```python
from build123d import *

# Parameters (mm, degrees)
SKETCH1_R           = 68.659375
SKETCH1_R_2         = 55.959375
BOSS_EXTRUDE1_DEPTH = 3.175
BOSS_EXTRUDE2_START = -3.175
BOSS_EXTRUDE2_DEPTH = 3.175
CIRPATTERN1_COUNT   = 9
SKETCH3_R           = 2.2225
CUT_EXTRUDE6_DEPTH  = 124.199501286
CIRPATTERN10_COUNT  = 9
CUT_EXTRUDE7_DEPTH  = 124.199501286
CIRPATTERN12_COUNT  = 9
FILLET1_R           = 5.08


with BuildPart() as part:
    # Sketch1 → Boss-Extrude1 (new body)
    with BuildSketch(Plane(origin=(0, 0, 0), x_dir=(1, 0, 0), z_dir=(0, 1, 0))):
        with Locations(Location((0, 0, 0), (0, 0, 270))):
            Circle(SKETCH1_R)
        with Locations(Location((0, 0, 0), (0, 0, 270))):
            Circle(SKETCH1_R_2, mode=Mode.SUBTRACT)
    extrude(amount=BOSS_EXTRUDE1_DEPTH)

    # Sketch2 → Boss-Extrude2 (add)
    with BuildSketch(Plane(origin=(0, 3.175, 0), x_dir=(1, 0, 0), z_dir=(0, 1, 0)).offset(BOSS_EXTRUDE2_START)):
        with BuildLine():
            Line((-4.653697789, 71.001707707), (-5.372788209, 81.972907412))
            ThreePointArc((-5.372788209, 81.972907412), (0, 87.709375), (5.372788209, 81.972907412))
            ThreePointArc((5.372788209, 81.972907412), (1.580107525, 80.725221164), (0.983574692, 76.777399446))
            Line((0.983574692, 76.777399446), (3.889375, 69.933810414))
            ThreePointArc((3.889375, 69.933810414), (4.734169071, 68.871766239), (6.005193091, 68.39625305))
            ThreePointArc((6.005193091, 68.39625305), (-0.46538454, 68.657797755), (-6.931822104, 68.308561818))
            ThreePointArc((-6.931822104, 68.308561818), (-5.249012804, 69.195180628), (-4.653697789, 71.001707707))
        make_face()
    boss_extrude2 = extrude(amount=BOSS_EXTRUDE2_DEPTH)

    # CirPattern1: Boss-Extrude2 ×9 about axis
    cirpattern1_axis = Axis((0, 0, 0), (0, 1, 0))
    for i in range(1, CIRPATTERN1_COUNT):
        add(boss_extrude2.rotate(cirpattern1_axis, i * 360 / CIRPATTERN1_COUNT))

    # Sketch3 → Cut-Extrude6 (cut, through all)
    with BuildSketch(Plane(origin=(0, 3.175, 0), x_dir=(1, 0, 0), z_dir=(0, 1, 0))):
        with Locations(Location((0, 84.132166, 0), (0, 0, 270))):
            Circle(SKETCH3_R)
    cut_extrude6 = extrude(amount=-CUT_EXTRUDE6_DEPTH, mode=Mode.SUBTRACT)

    # CirPattern10: Cut-Extrude6 ×9 about axis
    cirpattern10_axis = Axis((0, 0, 0), (0, 1, 0))
    for i in range(1, CIRPATTERN10_COUNT):
        add(cut_extrude6.rotate(cirpattern10_axis, i * 360 / CIRPATTERN10_COUNT), mode=Mode.SUBTRACT)

    # Sketch4 → Cut-Extrude7 (cut, through all)
    with BuildSketch(Plane(origin=(0, 3.175, 0), x_dir=(1, 0, 0), z_dir=(0, 1, 0))):
        with BuildLine():
            Line((18.267202623, 60.462203187), (6.005193091, 68.39625305))
            ThreePointArc((6.005193091, 68.39625305), (23.04503141, 64.676396797), (38.597813369, 56.78308356))
            Line((38.597813369, 56.78308356), (24.870866002, 58.05866628))
            ThreePointArc((24.870866002, 58.05866628), (21.122906044, 58.034707389), (18.267202623, 60.462203187))
        make_face()
    cut_extrude7 = extrude(amount=-CUT_EXTRUDE7_DEPTH, mode=Mode.SUBTRACT)

    # CirPattern12: Cut-Extrude7 ×9 about axis
    cirpattern12_axis = Axis((0, 0, 0), (0, 1, 0))
    for i in range(1, CIRPATTERN12_COUNT):
        add(cut_extrude7.rotate(cirpattern12_axis, i * 360 / CIRPATTERN12_COUNT), mode=Mode.SUBTRACT)

    # Fillet1
    fillet1_edges = [part.edges().sort_by_distance(p)[0] for p in [
        (-16.849122023, 1.5875, 66.559874267),
        (-62.235489211, 1.5875, 28.997476754),
        (-55.691038779, 1.5875, 40.157414946),
        (6.005193091, 1.5875, -68.39625305),
        (-66.314369444, 1.5875, -17.790845415),
        (-68.474499552, 1.5875, -5.035145128),
        (-6.931822104, 1.5875, -68.308561818),
        (-39.364019213, 1.5875, -56.254633292),
        (-49.217980976, 1.5875, -47.871704837),
        (24.870866002, 1.5875, -58.05866628),
        (18.267202623, 1.5875, -60.462203187),
        (56.371580016, 1.5875, -28.48883417),
        (52.857844124, 1.5875, -34.574803261),
        (61.49540524, 1.5875, 14.411240066),
        (62.715712909, 1.5875, 7.490531368),
        (37.844846907, 1.5875, 50.568134912),
        (43.228202617, 1.5875, 46.050963121),
        (-3.513735893, 1.5875, 63.063637431),
        (3.513735893, 1.5875, 63.063637431),
        (-43.228202617, 1.5875, 46.050963121),
        (-37.844846907, 1.5875, 50.568134912),
        (-62.715712909, 1.5875, 7.490531368),
        (-61.49540524, 1.5875, 14.411240066),
        (-52.857844124, 1.5875, -34.574803261),
        (-56.371580016, 1.5875, -28.48883417),
        (-18.267202623, 1.5875, -60.462203187),
        (-24.870866002, 1.5875, -58.05866628),
        (48.564508807, 1.5875, -48.534505867),
        (38.597813369, 1.5875, -56.78308356),
        (68.399951118, 1.5875, -5.962923987),
        (66.067103, 1.5875, -18.68816943),
        (56.23029612, 1.5875, 39.398776296),
        (62.622860883, 1.5875, 28.151146872),
        (17.749860638, 1.5875, 66.325351282),
        (29.876686184, 1.5875, 61.818228688),
        (-29.035931905, 1.5875, 62.217557279),
    ]]
    fillet(fillet1_edges, radius=FILLET1_R)


solid = part.part
```
Here's how the part is built. I have some questions about the finished solid (model axes, mm). A direction names the side the tool comes from. Coordinates: 2 decimals unless noted, no trailing zeros. Loops run counter-clockwise (first coordinate to the right, second up) from the corner with the lowest first, then second, coordinate; pieces in that order, holes last. Notation, with made-up numbers: (51.5, 1) - (109.5, 1) arc R27 cw to (109.5, 39) - close; hole circle Ø3 at (29, -32). An arc over 180 degrees is marked (long way). Return JSON: item names as keys, results as strings. Group by question number.
Item 1: On a 3-axis mill with a long thin cutter (end or side, diameter ignored), from which of +Z, -Z, +X, -X, +Y, -Y can I reach the whole of each face in a straight line? I mean faces 1 (the face through (-65.636, 1.61, 1.139)), 2 (the face through (30.84, 1.57, 70.09)), 3 (the face through (22.835, 1.565, 69.803)), 4 (the face through (45.279, 1.565, -61.753)). Say none if no direction works.
Item 2: If we section it at B-B on y = 2.25: State how many separate pieces and enclosed holes the cut face has, and give its area (3 significant figures).
Item 3: Will this pin go through, and if not, where does the flat tip stop? P1, Ø1.5, axis at y = 0.5, z = -42, coming from the -X side.
Item 4: If we section it at A-A on z = 0: Write out the boundary of the cut face in (x, y) (3 decimals).
Item 5: If we section it at C-C on z = -25.5: Write out the boundary of the cut face in (x, y) (3 decimals), and give its area (3 significant figures).
Item 6: I need wall thicknesses on line 1 (Z direction, x = 25.5, y = 2.7); line 2 (X direction, y = 0.6, z = -14); line 3 (X direction, y = 0.9, z = 42.5). Which ranges of each line are inside material? Lowest first, please. Write a range as from..to.
Item 7: We'd pull the mould along X, two halves only. Please class faces 5 (the face through (39.65, 1.61, 47.35)), 6 (the face through (-38, 0, 41.3)), 7 (the face through (50.72, 1.61, -41.53)): +X half, -X half, draft (parallel to the pull), parting line (faces both ways), or undercut.
Calculated:
{
 "1": {"face 1": "-X, +Y, -Y", "face 2": "+X, +Y, -Y", "face 3": "+Y, -Y", "face 4": "-Z, +Y, -Y"},
 "2": {"separate pieces": "1", "enclosed holes": "10", "area": "4,990 mm^2"},
 "3": {"P1": "stops at x = -51.03"},
 "4": {"outline": "(-66.16, 0) - (-55.959, 0) - (-55.959, 3.175) - (-66.16, 3.175) - close; (55.959, 0) - (65.881, 0) - (65.881, 3.175) - (55.959, 3.175) - close"},
 "5": {"outline": "(-59.149, 0) - (-49.812, 0) - (-49.812, 3.175) - (-59.149, 3.175) - close; (49.812, 0) - (59.328, 0) - (59.328, 3.175) - (49.812, 3.175) - close", "area": "59.9 mm^2"},
 "6": {"line 1": "z = -57.99..-49.81, 49.81..72.67, 77.49..82.04", "line 2": "x = -86.45..-84.99, -80.72..-54.18, 54.18..80.72, 84.99..86.45", "line 3": "x = -76.51..-75.04, -70.68..-63.61, -50.74..-36.4, 36.4..50.17, 69.31..70.68, 75.04..76.51"},
 "7": {"face 5": "undercut", "face 6": "draft", "face 7": "+X half"}
}
